Can you work these out from the model? Positions are in its coordinate system, mm. Coordinates: 2 decimals unless noted, no trailing zeros. Answer as a JSON object with one key per item and string values. Group by question number.
(1) I need wall thicknesses on line 1 (X direction, y = -25.5, z = -1.4); line 2 (Y direction, x = 25.4, z = 0.5). Which ranges of each line are inside material? Lowest first, please.
(2) I want a section at A-A, the plane y = -25.4. State how many separate pieces and enclosed holes the cut face has, plus the area to 3 significant figures.
(3) If we mould it in two halves opening along Y, with no side actions, what happens to faces 1 (the cylindrical face through (1.755, 2.752, 0.028)), 2 (the flat face through (1, -38.1, 0)), 3 (the cylindrical face through (25.562, 12.205, -2.315)), 4 (the flat face through (38.1, -25, 0))? For each: pulls with the +Y half, pulls with the -Y half, needs draft (parallel to the pull), parting line crosses it, or undercut.
(4) For pin 1 (2 mm diameter, centred on x = -13.5, z = -2, fed in from +Y); pin 2 (1 mm diameter, centred on x = 27.5, z = 2, fed in from +Y); pin 3 (2 mm diameter, centred on y = 18, z = -2, fed in from -X), each with a flat end and sliding along its axis, tell me the tip position at first contact or that it passes through.
from build123d import *

# Parameters (mm, degrees)
BOSS_EXTRUDE1_START        = -2.3876
BOSS_EXTRUDE1_DEPTH        = 4.7752
SKETCH4_R                  = 3.2639
CUT_EXTRUDE1_DEPTH         = 55.092721646
CHAMFER1_SIZE              = 0.381
LPATTERN1_COUNT            = 3
LPATTERN1_PITCH            = 25.4
LPATTERN1_COUNT_DIR2       = 3
LPATTERN1_PITCH_DIR2       = 25.4
CHAMFER1_OF_LPATTERN1_SIZE = 0.381
FILLET1_R                  = 0.635
FILLET2_R                  = 0.254


with BuildPart() as part:
    # Sketch3 → Boss-Extrude1 (new body)
    with BuildSketch(Plane.XY.offset(BOSS_EXTRUDE1_START)):
        Polygon((-38.1, -38.1), (-38.1, -12.7), (-12.7, 38.1), (12.7, 38.1), (38.1, -12.7), (38.1, -38.1), align=None)
    extrude(amount=BOSS_EXTRUDE1_DEPTH)

    # Sketch4 → Cut-Extrude1 (cut, through all)
    with BuildSketch(Plane.XY.offset(2.3876)):
        with Locations((-25.4, -25.4)):
            Circle(SKETCH4_R)
    cut_extrude1 = extrude(amount=-CUT_EXTRUDE1_DEPTH, mode=Mode.SUBTRACT)

    # Chamfer1
    chamfer1_edges = [part.edges().sort_by_distance(p)[0] for p in [
        (-28.6639, -25.4, -2.3876),
        (-28.6639, -25.4, 2.3876),
    ]]
    chamfer(chamfer1_edges, length=CHAMFER1_SIZE)

    # LPattern1: Cut-Extrude1 3 × 3, 4 skipped
    with Locations(*[(i * LPATTERN1_PITCH, j * LPATTERN1_PITCH_DIR2, 0) for i in range(LPATTERN1_COUNT) for j in range(LPATTERN1_COUNT_DIR2) if (i, j) not in ((0, 0), (0, 1), (0, 2), (2, 1), (2, 2))]):
        add(cut_extrude1, mode=Mode.SUBTRACT)

    # Chamfer1 of LPattern1
    chamfer1_of_lpattern1_edges = [part.edges().sort_by_distance(p)[0] for p in [
        (-3.2639, -25.4, -2.3876),
        (-3.2639, -25.4, 2.3876),
        (-3.2639, 0, -2.3876),
        (-3.2639, 0, 2.3876),
        (-3.2639, 25.4, -2.3876),
        (-3.2639, 25.4, 2.3876),
        (22.1361, -25.4, -2.3876),
        (22.1361, -25.4, 2.3876),
    ]]
    chamfer(chamfer1_of_lpattern1_edges, length=CHAMFER1_OF_LPATTERN1_SIZE)

    # Fillet1
    fillet1_edges = [part.edges().sort_by_distance(p)[0] for p in [
        (-38.1, -38.1, 0),
        (-38.1, -12.7, 0),
        (-12.7, 38.1, 0),
        (12.7, 38.1, 0),
        (38.1, -12.7, 0),
        (38.1, -38.1, 0),
    ]]
    fillet(fillet1_edges, radius=FILLET1_R)

    # Fillet2
    fillet2_edges = [part.edges().sort_by_distance(p)[0] for p in [
        (0, -38.1, -2.3876),
        (0, -38.1, 2.3876),
        (-38.1, -25.157451583, -2.3876),
        (-25.454235475, 12.59152905, -2.3876),
        (0, 38.1, -2.3876),
        (25.454235475, 12.59152905, -2.3876),
        (38.1, -25.157451583, -2.3876),
        (38.083013108, -12.704010061, -2.3876),
        (37.914012806, -37.914012806, -2.3876),
        (12.641387673, 38.005163263, -2.3876),
        (-12.641387673, 38.005163263, -2.3876),
        (-38.083013108, -12.704010061, -2.3876),
        (-37.914012806, -37.914012806, -2.3876),
        (-38.1, -25.157451583, 2.3876),
        (38.1, -25.157451583, 2.3876),
        (25.454235475, 12.59152905, 2.3876),
        (0, 38.1, 2.3876),
        (-25.454235475, 12.59152905, 2.3876),
        (38.083013108, -12.704010061, 2.3876),
        (37.914012806, -37.914012806, 2.3876),
        (12.641387673, 38.005163263, 2.3876),
        (-12.641387673, 38.005163263, 2.3876),
        (-38.083013108, -12.704010061, 2.3876),
        (-37.914012806, -37.914012806, 2.3876),
    ]]
    fillet(fillet2_edges, radius=FILLET2_R)


solid = part.part
Computed values:
{
 "1": {"line 1": "x = -38.1 to -28.66, -22.14 to -3.26, 3.26 to 22.14, 28.66 to 38.1", "line 2": "y = -38.1 to -28.66, -22.14 to 12.7"},
 "2": {"separate pieces": "4", "enclosed holes": "0", "area": "269 mm2"},
 "3": {"face 1": "undercut", "face 2": "pulls with the -Y half", "face 3": "pulls with the +Y half", "face 4": "needs draft"},
 "4": {"pin 1": "stops at y = 38.07", "pin 2": "stops at y = 9.5", "pin 3": "stops at x = -23.25"}
}
